```python
from build123d import *

# Parameters (mm, degrees)
F1_DEPTH  = 35
F2_W      = 14
F2_H      = 80
F3_DEPTH  = 15
F4_R      = 32.5
F5_DEPTH  = 15
F6_W      = 14
F6_H      = 66.9722852701
F7_DEPTH  = 20
F8_DEPTH  = 5
F9_R      = 5
F11_DEPTH = 15


with BuildPart() as f1:
    # F0 (on Right) → F1 (new body)
    with BuildSketch(Plane.YZ):
        with BuildLine():
            Line((58.0277147299, 59.5856680407), (-111.9722852701, 59.5856680407))
            ThreePointArc((-111.9722852701, 59.5856680407), (-115.507819176, 58.1212019466), (-116.9722852701, 54.5856680407))
            Line((-116.9722852701, 54.5856680407), (-116.9722852701, -35.4143319593))
            ThreePointArc((-116.9722852701, -35.4143319593), (-115.507819176, -38.9498658653), (-111.9722852701, -40.4143319593))
            Line((-111.9722852701, -40.4143319593), (58.0277147299, -40.4143319593))
            ThreePointArc((58.0277147299, -40.4143319593), (61.5632486359, -38.9498658653), (63.0277147299, -35.4143319593))
            Line((63.0277147299, -35.4143319593), (63.0277147299, 54.5856680407))
            ThreePointArc((63.0277147299, 54.5856680407), (61.5632486359, 58.1212019466), (58.0277147299, 59.5856680407))
        make_face()
    extrude(amount=F1_DEPTH)

    # F2 (on face) → F3 (cut)
    with BuildSketch(Plane.XY.offset(59.5856680407)):
        with Locations((7, -26.9722852701)):
            Rectangle(F2_W, F2_H)
    extrude(amount=-F3_DEPTH, mode=Mode.SUBTRACT)

    # F4 (on face) → F5 (cut)
    with BuildSketch(Plane(origin=(0, 0, 0), x_dir=(0, -1, 0), z_dir=(-1, 0, 0))):
        with Locations((26.9722852701, 0)):
            Circle(F4_R)
    extrude(amount=-F5_DEPTH, mode=Mode.SUBTRACT)

    # F6 (on face) → F7 (cut)
    with BuildSketch(Plane.XY.offset(59.5856680407)):
        with Locations((7, -33.486142635)):
            Rectangle(F6_W, F6_H)
    extrude(amount=-F7_DEPTH, mode=Mode.SUBTRACT)

    # F8 (cut): a face of the model
    f8_faces = [f1.faces().sort_by_distance(p)[0] for p in [
        (7, 6.513857365, 44.5856680407),
    ]]
    extrude(f8_faces, amount=-F8_DEPTH, mode=Mode.SUBTRACT)

    # F9
    f9_edges = [f1.edges().sort_by_distance(p)[0] for p in [
        (35, 61.563249, 58.121202),
        (35, -26.972285, 59.585668),
        (35, -115.507819, 58.121202),
        (35, -116.972285, 9.585668),
        (35, -115.507819, -38.949866),
        (35, -26.972285, -40.414332),
        (35, 61.563249, -38.949866),
        (35, 63.027715, 9.585668),
    ]]
    fillet(f9_edges, radius=F9_R)

    # F10 (on face) → F11 (cut)
    with BuildSketch(Plane(origin=(0, 0, 0), x_dir=(0, -1, 0), z_dir=(-1, 0, 0))):
        with BuildLine():
            Line((100.1400923047, 1.4106337988), (66.9722852701, 39.5856680407))
            Line((66.9722852701, 39.5856680407), (46.274099499, 39.5856680407))
            Line((46.274099499, 39.5856680407), (79.0167047111, 10.1334832275))
            ThreePointArc((79.0167047111, 10.1334832275), (80.3412411164, 4.6254181345), (75.672894817, 1.4161003589))
            Line((75.672894817, 1.4161003589), (59.4414192248, 1.4161003589))
            ThreePointArc((59.4414192248, 1.4161003589), (59.4645678425, 0.7082183525), (59.4722852701, 0))
            ThreePointArc((59.4722852701, 0), (58.8613058145, -6.2721901054), (57.0513395028, -12.3085537925))
            Line((57.0513395028, -12.3085537925), (96.3657003641, -12.3085537925))
            ThreePointArc((96.3657003641, -12.3085537925), (99.90123427, -10.8440876985), (101.3657003641, -7.3085537925))
            Line((101.3657003641, -7.3085537925), (101.3657003641, -1.8686901374))
            ThreePointArc((101.3657003641, -1.8686901374), (101.049286581, -0.1182558632), (100.1400923047, 1.4106337988))
        make_face()
    extrude(amount=-F11_DEPTH, mode=Mode.SUBTRACT)


solid = f1.part
```
Here's how the part is built. I have some questions about the finished solid (model axes, mm). A direction names the side the tool comes from. Give positions to 0.01 mm unless a question says otherwise; leave off trailing zeros. Write each loop counter-clockwise with the first axis right and the second up, starting at its lowest first coordinate (ties: lowest second). Pieces come first, ordered by that corner, then holes.
(1) If I drill on L1, parallel to X at y = -16.5, z = 7; L2, parallel to Z at x = 10, y = -43; L3, parallel to Y at x = 3.25, z = 0, over which ranges is the centre line in solid material (lowest first)?
Output values:
L1: x = 15 to 35
L2: z = -40.41 to -28.27, 28.27 to 39.59
L3: y = -116.97 to -101, 5.53 to 63.03
(2) Imagine slicing it at A-A, the plane x = 6. Write out the boundary of the cut face in (y, z).
Output values:
outline: (-116.97, -35.41) arc R5 ccw to (-111.97, -40.41) - (58.03, -40.41) arc R5 ccw to (63.03, -35.41) - (63.03, 54.59) arc R5 ccw to (58.03, 59.59) - (13.03, 59.59) - (13.03, 39.59) - (-46.27, 39.59) - (-79.02, 10.13) arc R5 ccw to (-75.67, 1.42) - (-59.44, 1.42) arc R32.5 cw (long way) to (-57.05, -12.31) - (-96.37, -12.31) arc R5 cw to (-101.37, -7.31) - (-101.37, -1.87) arc R5 cw to (-100.14, 1.41) - (-66.97, 39.59) - (-66.97, 59.59) - (-111.97, 59.59) arc R5 ccw to (-116.97, 54.59) - close
(3) Thinking about a two-plate mould opening in Z: for faces 4 (the face through (14.79, -115.55, -38.91)), 5 (the face through (15, 63.028, 9)), 6 (the face through (7.395, -99.862, -10.883)), which applies, pulls with the +Z half, pulls with the -Z half, needs draft (parallel to the pull), parting line crosses it, or undercut?
Output values:
face 4: pulls with the -Z half
face 5: needs draft
face 6: undercut
(4) Imagine slicing it at C-C, the plane y = -53. Write out the boundary of the cut face in (x, z), and give its area (3 significant figures).
Output values:
outline: (0, -40.41) - (30, -40.41) arc R5 ccw to (35, -35.41) - (35, 54.59) arc R5 ccw to (30, 59.59) - (14, 59.59) - (14, 39.59) - (15, 39.59) - (15, 33.54) - (0, 33.54) - (0, 19.46) - (15, 19.46) - (15, -19.46) - (0, -19.46) - close
area: 2,530 mm2
(5) On a 3-axis mill with a long thin cutter (end or side, diameter ignored), from which of +Z, -Z, +X, -X, +Y, -Y can I reach the whole of each face in a straight line? I mean faces 1 (the face through (7.4, 4.79, 6.88)), 2 (the face through (7, 13.028, 50)), 3 (the face through (14.79, -115.47, 58.16)). Say none if no direction works.
Output values:
face 1: -X
face 2: +Z, -X
face 3: +Z, +X, -X, -Y
(6) Will this pin go through, and if not, where does the flat tip stop? pin 1 (7 mm diameter, centred on x = 5, y = -28, fed in from +Z).
Output values:
pin 1: stops at z = 39.59
(7) Imagine slicing it at B-B, the plane z = -14. Write out the boundary of the cut face in (x, y), and give its area (3 significant figures).
Output values:
outline: (0, -116.97) - (30, -116.97) arc R5 ccw to (35, -111.97) - (35, 58.03) arc R5 ccw to (30, 63.03) - (0, 63.03) - (0, 2.36) - (15, 2.36) - (15, -56.3) - (0, -56.3) - close
area: 5,410 mm2
(8) Imagine slicing it at D-D, the plane z = 35. Write out the boundary of the cut face in (x, y), and give its area (3 significant figures).
Output values:
outline: (0, -116.97) - (30, -116.97) arc R5 ccw to (35, -111.97) - (35, 58.03) arc R5 ccw to (30, 63.03) - (0, 63.03) - (0, -51.37) - (15, -51.37) - (15, -70.96) - (0, -70.96) - close
area: 6,000 mm2
